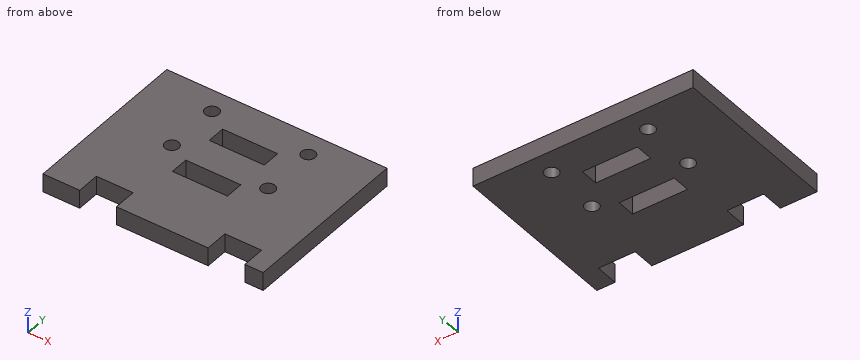
```python
from build123d import *

# Parameters (mm, degrees)
SKETCH1_R           = 0.75
SKETCH1_W           = 6
SKETCH1_H           = 2
BOSS_EXTRUDE1_DEPTH = 2


with BuildPart() as part:
    # Sketch1 → Boss-Extrude1 (new body)
    with BuildSketch(Plane.XY):
        Polygon((5, 2), (9, 2), (9, -0.5), (19, -0.5), (19, 2), (23, 2), (23, -0.5), (25, -0.5), (25, 18), (1, 18), (1, -0.5), (5, -0.5), align=None)
        with Locations((7.75, 15.5)):
            Circle(SKETCH1_R, mode=Mode.SUBTRACT)
        with Locations((18.25, 15.5)):
            Circle(SKETCH1_R, mode=Mode.SUBTRACT)
        with Locations((18.25, 9.5)):
            Circle(SKETCH1_R, mode=Mode.SUBTRACT)
        with Locations((7.75, 9.5)):
            Circle(SKETCH1_R, mode=Mode.SUBTRACT)
        with Locations((13, 13)):
            Rectangle(SKETCH1_W, SKETCH1_H, mode=Mode.SUBTRACT)
        with Locations((13, 7.5)):
            Rectangle(SKETCH1_W, SKETCH1_H, mode=Mode.SUBTRACT)
    extrude(amount=BOSS_EXTRUDE1_DEPTH)


solid = part.part
```
Check sheet for the modelled part. Datum: model origin and axes. Units: mm. Coordinates: 2 decimals unless noted, no trailing zeros. Order: outer loops, then holes, each group sorted by start corner. A loop starts at its lowest first (then second) coordinate and runs counter-clockwise, first axis right, second up. Notation, with made-up numbers: (-34.75, 63.5) -> (1.25, 63.5) arc R30 cw to (1.25, 94.5) -> close; hole circle Ø2 at (40, 72.5). An arc over 180 degrees is marked (long way). Write item = value, one per line. Start each with the question number.
1) Go/stop test with a flat-tipped pin: P1, Ø1, axis at x = 8, z = 1, coming from the -Y side. Record where the tip stops, or that it passes through.
2) Material ranges on L1, parallel to Y at x = 14.25, z = 0.8; L2, parallel to Y at x = 7.75, z = 1.65; L3, parallel to X at y = 13, z = 1.2, recorded low to high.
3) Cross-section at A-A (x = 7.75). Enter the section's corners in (y, z), then the cut area to 3 significant figures.
4) Cross-section at C-C (y = 15.5). Enter the section's corners in (x, z).
5) Cross-section at D-D (y = 7.25). Enter the section's corners in (x, z).
6) Cross-section at B-B (z = 1.05). Enter the section's corners in (x, y).
Ans:
q1.P1 = 2
q2.L1 = -0.5 to 6.5, 8.5 to 12, 14 to 18
q2.L2 = 2 to 8.75, 10.25 to 14.75, 16.25 to 18
q2.L3 = 1 to 10, 16 to 25
q3.outline = (2, 0) -> (8.75, 0) -> (8.75, 2) -> (2, 2) -> close; (10.25, 0) -> (14.75, 0) -> (14.75, 2) -> (10.25, 2) -> close; (16.25, 0) -> (18, 0) -> (18, 2) -> (16.25, 2) -> close
q3.area = 26.0 mm²
q4.outline = (1, 0) -> (7, 0) -> (7, 2) -> (1, 2) -> close; (8.5, 0) -> (17.5, 0) -> (17.5, 2) -> (8.5, 2) -> close; (19, 0) -> (25, 0) -> (25, 2) -> (19, 2) -> close
q5.outline = (1, 0) -> (10, 0) -> (10, 2) -> (1, 2) -> close; (16, 0) -> (25, 0) -> (25, 2) -> (16, 2) -> close
q6.outline = (1, -0.5) -> (5, -0.5) -> (5, 2) -> (9, 2) -> (9, -0.5) -> (19, -0.5) -> (19, 2) -> (23, 2) -> (23, -0.5) -> (25, -0.5) -> (25, 18) -> (1, 18) -> close; hole circle Ø1.5 at (7.75, 9.5); hole circle Ø1.5 at (7.75, 15.5); hole (10, 6.5) -> (16, 6.5) -> (16, 8.5) -> (10, 8.5) -> close; hole (10, 12) -> (16, 12) -> (16, 14) -> (10, 14) -> close; hole circle Ø1.5 at (18.25, 9.5); hole circle Ø1.5 at (18.25, 15.5)
